Job drawing, mm, ordinate dimensions from the low corner. One solid piece. A direction names the side the tool comes from. Round coordinates to 2 decimals unless told otherwise and drop trailing zeros. Loops run counter-clockwise (first coordinate to the right, second up) from the corner with the lowest first, then second, coordinate; pieces in that order, holes last. Notation, with made-up numbers: M 8.5,47.5 L 54.5,47.5 A21 cw 54.5,83.5 Z; hole C -34.75,38.25 d3. An arc over 180 degrees is marked long. Use a Markdown table: item, result. Add a question column.
(1) Band-saw the part on A-A, the plane y = 30.5. Write the cut outline in (x, z).
(2) Which spindle directions (+Z, -Z, +X, -X, +Y, -Y) get a long thin tool onto all of the face, cutting with end or side? Do the marked faces 4 and 5. Say none if no direction does.
(3) Two-plate mould, pull along Y, no slides. Class the marked faces 1, 2 and 3: released by +Y, released by -Y, zero draft, split by the parting line, or undercut.
(4) Flat gauge pins, fed straight in: P1, Ø0.6, axis at x = 30.5, z = 28.5, coming from the +Y side; P2, Ø1.5, axis at x = 22, z = 18, coming from the -Y side; P3, Ø20, axis at x = 19, z = 28, coming from the -Y side. Where does each tip first touch, or does it go through?
(5) Band-saw the part on B-B, the plane x = 19.5. Write the cut outline in (y, z).
(6) Wall check: L1, parallel to Y at x = 19, z = 12.5 (1 decimal); L2, parallel to X at y = 23.5, z = 31; L3, parallel to X at y = 66.5, z = 15. Give the ranges that are in metal, low to high.
(7) Band-saw the part on D-D, the plane y = 113.5. Write the cut outline in (x, z).
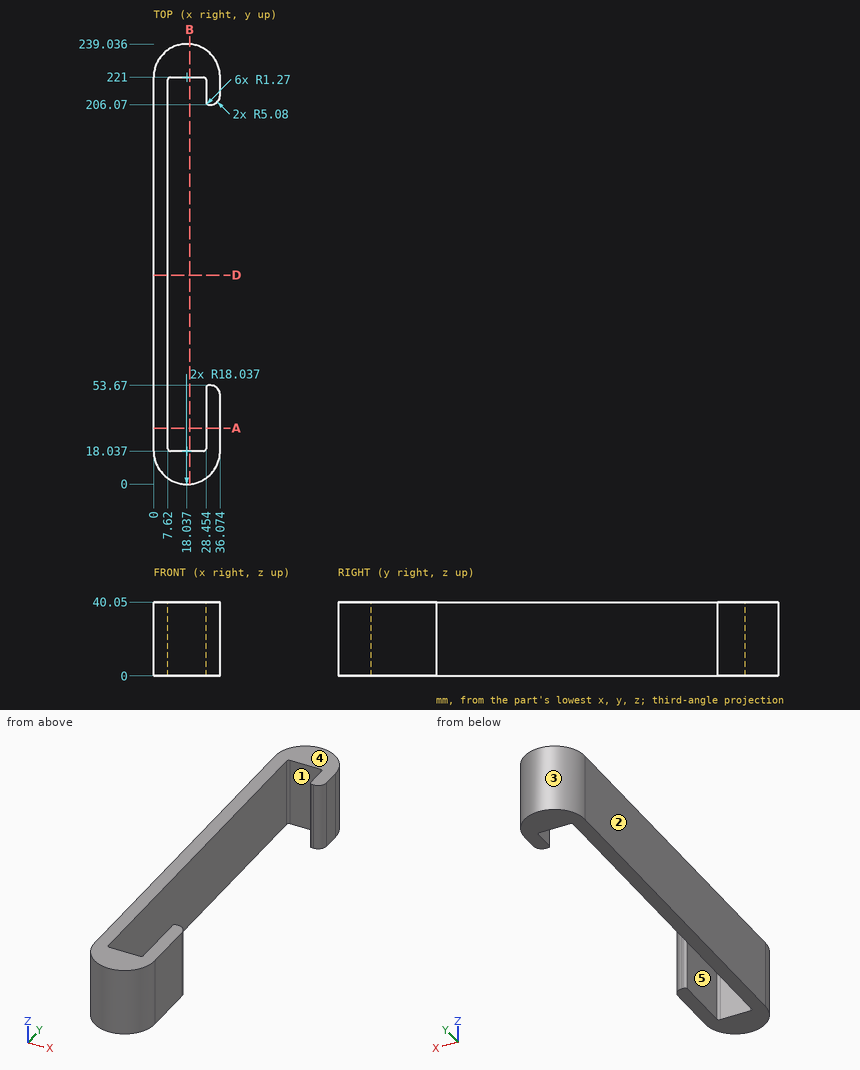
Return value:
| question | item | result |
|---|---|---|
| 1 | outline | M 0,0 L 7.62,0 L 7.62,40.05 L 0,40.05 Z; M 28.45,0 L 36.07,0 L 36.07,40.05 L 28.45,40.05 Z |
| 2 | face 4 | +Z, +X, -X, +Y, -Y |
| 2 | face 5 | +Z, -Z |
| 3 | face 1 | undercut |
| 3 | face 2 | zero draft |
| 3 | face 3 | released by +Y |
| 4 | P1 | y = 234.32 |
| 4 | P2 | y = 0.29 |
| 4 | P3 | y = 0 |
| 5 | outline | M 0.06,0 L 18.04,0 L 18.04,40.05 L 0.06,40.05 Z; M 221,0 L 238.98,0 L 238.98,40.05 L 221,40.05 Z |
| 6 | L1 | 0 to 18, 221 to 239 |
| 6 | L2 | 0 to 7.62, 28.45 to 36.07 |
| 6 | L3 | 0 to 7.62 |
| 7 | outline | M 0,0 L 7.62,0 L 7.62,40.05 L 0,40.05 Z |
